```python
from build123d import *

# Parameters (mm, degrees)
F0_W     = 50
F0_H     = 50
F0_W_2   = 40
F0_H_2   = 40
F1_DEPTH = 520
F2_R     = 5
F3_R     = 3
F5_D     = 10.5


with BuildPart() as f1:
    # F0 (on Front) → F1 (new body)
    with BuildSketch(Plane.XZ):
        Rectangle(F0_W, F0_H)
        Rectangle(F0_W_2, F0_H_2, mode=Mode.SUBTRACT)
    extrude(amount=F1_DEPTH)

    # F2
    f2_edges = [f1.edges().sort_by_distance(p)[0] for p in [
        (25, -260, 25),
        (-25, -260, 25),
        (25, -260, -25),
        (-25, -260, -25),
    ]]
    fillet(f2_edges, radius=F2_R)

    # F3
    f3_edges = [f1.edges().sort_by_distance(p)[0] for p in [
        (-20, -260, 20),
        (20, -260, 20),
        (20, -260, -20),
        (-20, -260, -20),
    ]]
    fillet(f3_edges, radius=F3_R)

    # F5 (through all)
    with Locations(Plane(origin=(0, 0, -25), x_dir=(1, 0, 0), z_dir=(0, 0, -1))):
        with Locations((0, 15)):
            Hole(F5_D / 2)


solid = f1.part
```
Work out the finished part from the listing and answer in its coordinate system (mm). A direction names the side the tool comes from. Give positions to 0.01 mm unless a question says otherwise; leave off trailing zeros. Order: outer loops, then holes, each group sorted by start corner. A loop starts at its lowest first (then second) coordinate and runs counter-clockwise, first axis right, second up. Notation, with made-up numbers: M 73,43 L 87,43 A17 cw 87,51 Z; hole C 39,24 d6. An arc over 180 degrees is marked long. Return JSON: item names as keys, results as strings.
1) Section C-C, the plane x = 0 is taken. Write down the section's boundary in (y, z), plus the area to 4 significant figures.
Resolved:
{"outline": "M -520,-25 L -20.25,-25 L -20.25,-20 L -520,-20 Z; M -520,20 L -20.25,20 L -20.25,25 L -520,25 Z; M -9.75,-25 L 0,-25 L 0,-20 L -9.75,-20 Z; M -9.75,20 L 0,20 L 0,25 L -9.75,25 Z", "area": "5,095 mm^2"}
2) Straight lines are drawn through the part: line 1 along Z through (x, y) = (-13.5, -392); line 2 along Y through (x, z) = (0, -21.9). For each, find the intervals that lie inside material, in ascending order. Write a range as [from, to].
Resolved:
{"line 1": "[-25, -20], [20, 25]", "line 2": "[-520, -20.25], [-9.75, 0]"}
3) Section A-A, the plane y = -120.5 is taken. Write down the section's boundary in (x, z).
Resolved:
{"outline": "M -25,-20 A5 ccw -20,-25 L 20,-25 A5 ccw 25,-20 L 25,20 A5 ccw 20,25 L -20,25 A5 ccw -25,20 Z; hole M -20,-17 A3 ccw -17,-20 L 17,-20 A3 ccw 20,-17 L 20,17 A3 ccw 17,20 L -17,20 A3 ccw -20,17 Z"}
4) Section D-D, the plane y = -15 is taken. Write down the section's boundary in (x, z), plus the area to 3 significant figures.
Resolved:
{"outline": "M -25,-20 A5 ccw -20,-25 L -5.25,-25 L -5.25,-20 L -17,-20 A3 cw -20,-17 L -20,17 A3 cw -17,20 L -5.25,20 L -5.25,25 L -20,25 A5 ccw -25,20 Z; M 5.25,-25 L 20,-25 A5 ccw 25,-20 L 25,20 A5 ccw 20,25 L 5.25,25 L 5.25,20 L 17,20 A3 cw 20,17 L 20,-17 A3 cw 17,-20 L 5.25,-20 Z", "area": "781 mm^2"}
5) Each of these flat-tipped pins is pushed along its axis until it touches: pin 1 (8.5 mm diameter, centred on x = 0, y = -15, fed in from +Z); pin 2 (10 mm diameter, centred on x = 20, z = -4, fed in from +Y). Where does it stop, or does it pass through?
Resolved:
{"pin 1": "through", "pin 2": "y = 0"}
6) Section B-B, the plane z = -7.5 is taken. Write down the section's boundary in (x, y), plus the area to 3 significant figures.
Resolved:
{"outline": "M -25,-520 L -20,-520 L -20,0 L -25,0 Z; M 20,-520 L 25,-520 L 25,0 L 20,0 Z", "area": "5,200 mm^2"}
7) For a pull along X with two mould halves and no side action, classify faces 1 (the flat face through (-25, -256, 0)), 2 (the flat face through (-23, -520, 0)), 3 (the flat face through (-20, -256, 0)) as +X half, -X half, draft (parallel to the pull), parting line (faces both ways), or undercut.
Resolved:
{"face 1": "-X half", "face 2": "draft", "face 3": "undercut"}
8) A tool of negligible diameter and unlimited length cuts with its end or side. For faces 4 (the flat face through (20, -256, 0)), 5 (the flat face through (0, -256, 25)), from which of +Z, -Z, +X, -X, +Y, -Y can it reach the whole face along a straight path? Write none if from no direction.
Resolved:
{"face 4": "+Y, -Y", "face 5": "+Z, +X, -X, +Y, -Y"}
